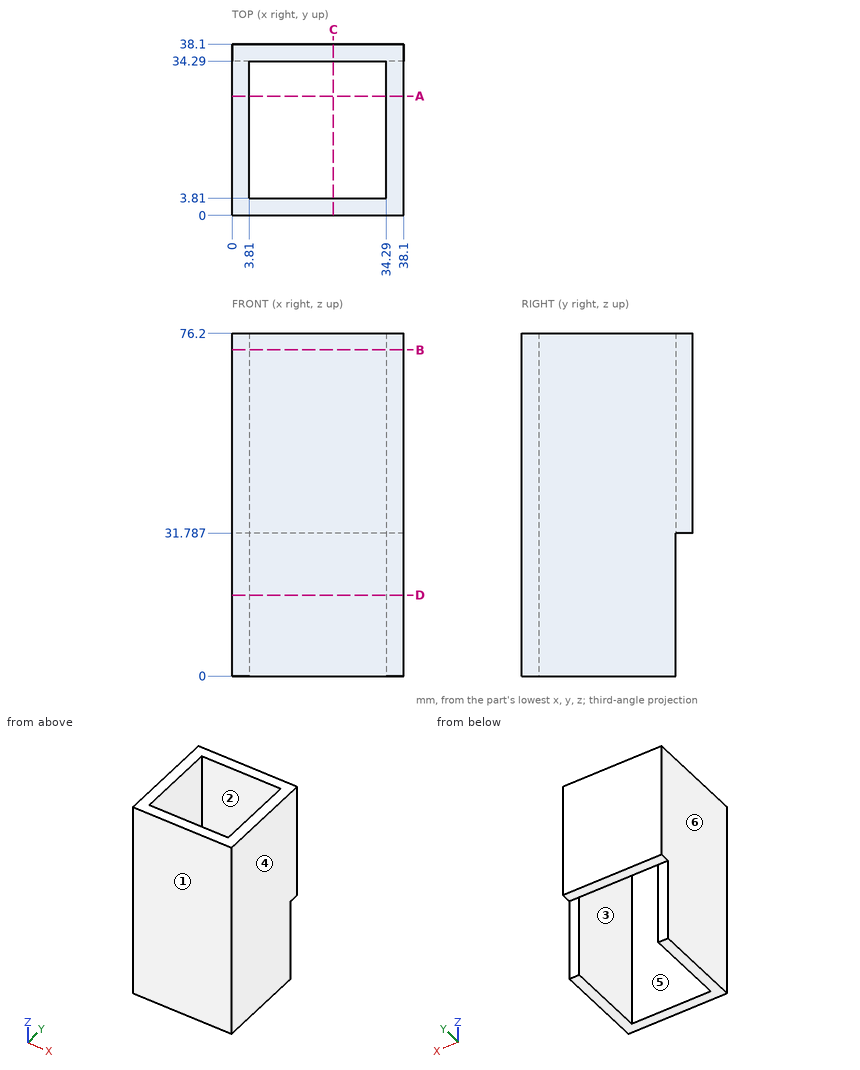
Study the drawing (mm; zero at the part's minimum x, y, z) and answer. A direction names the side the tool comes from. Round coordinates to 2 decimals unless told otherwise and drop trailing zeros. Write each loop counter-clockwise with the first axis right and the second up, starting at its lowest first coordinate (ties: lowest second). Pieces come first, ordered by that corner, then holes.
Q1. The mould has two halves that part along X. Classify the marked faces 1, 2, 3 and 4: released by +X, released by -X, zero draft, split by the parting line, or undercut.
Values:
face 1: zero draft
face 2: undercut
face 3: undercut
face 4: released by +X
Q2. Find section D-D on z = 18. Determine the outline of the cut face in (x, y).
Values:
outline: (0, 0) - (38.1, 0) - (38.1, 34.29) - (34.29, 34.29) - (34.29, 3.81) - (3.81, 3.81) - (3.81, 34.29) - (0, 34.29) - close
Q3. Flat-ended cylindrical pins translate along their axes: P1, Ø3, axis at x = 33, y = 23, coming from the -Z side; P2, Ø8, axis at x = 25.5, y = 30.5, coming from the -Z side; P3, Ø1.9, axis at x = 1, z = 21.5, coming from the +Y side. Find the tip coordinate at first contact, or state that the pin passes through.
Values:
P1: stops at z = 0
P2: stops at z = 31.79
P3: stops at y = 34.29
Q4. A tool of negligible diameter and unlimited length cuts with its end or side. For the marked faces 5 and 6, from which of +Z, -Z, +X, -X, +Y, -Y can it reach the whole face along a straight path? Write none if from no direction.
Values:
face 5: +Z, -Z
face 6: +Z, -Z, -X, +Y, -Y
Q5. Straight lines are drawn through the part: line 1 (X direction, y = 11, z = 4.5); line 2 (Y direction, x = 13.5, z = 28.5). For each, find the intervals that lie inside material, in ascending order.
Values:
line 1: x = 0 to 3.81, 34.29 to 38.1
line 2: y = 0 to 3.81
Q6. Find section C-C on x = 22.5. Determine the outline of the cut face in (y, z).
Values:
outline: (0, 0) - (3.81, 0) - (3.81, 76.2) - (0, 76.2) - close; (34.29, 31.79) - (38.1, 31.79) - (38.1, 76.2) - (34.29, 76.2) - close
Q7. Find section B-B on z = 72.5. Determine the outline of the cut face in (x, y).
Values:
outline: (0, 0) - (38.1, 0) - (38.1, 38.1) - (0, 38.1) - close; hole (3.81, 3.81) - (34.29, 3.81) - (34.29, 34.29) - (3.81, 34.29) - close
Q8. Find section A-A on y = 26.5. Determine the outline of the cut face in (x, z), and give its area (3 significant figures).
Values:
outline: (0, 0) - (3.81, 0) - (3.81, 76.2) - (0, 76.2) - close; (34.29, 0) - (38.1, 0) - (38.1, 76.2) - (34.29, 76.2) - close
area: 581 mm2
